Geometry: final body of the model. Coordinates: model frame, mm. Face numbers are marked on the shaded views. A direction names the side the tool comes from. Coordinates: 2 decimals unless noted, no trailing zeros. Order: outer loops, then holes, each group sorted by start corner. A loop starts at its lowest first (then second) coordinate and runs counter-clockwise, first axis right, second up. Notation, with made-up numbers: (47, -34.5) - (97, -34.5) arc R19 cw to (97, -13.5) - close; hole circle Ø1 at (62.5, -13). An arc over 180 degrees is marked (long way). Use a Markdown table: item, result. Add a question column.
```python
from build123d import *

# Parameters (mm, degrees)
F0_R     = 3.2385
F1_DEPTH = 6.35
F3_DEPTH = 4.318
F4_D     = 6.7564


with BuildPart() as f1:
    # F0 (on Top) → F1 (new body)
    with BuildSketch(Plane.XY):
        Polygon((0, -12.7), (10.9985226281, -6.35), (10.9985226281, 6.35), (0, 12.7), (-10.9985226281, 6.35), (-10.9985226281, -6.35), align=None)
        Polygon((0, 6.3204843369), (5.4737, 3.1602421685), (5.4737, -3.1602421685), (0, -6.3204843369), (-5.4737, -3.1602421685), (-5.4737, 3.1602421685), align=None, mode=Mode.SUBTRACT)
        Polygon((5.4737, -3.1602421685), (5.4737, 3.1602421685), (0, 6.3204843369), (-5.4737, 3.1602421685), (-5.4737, -3.1602421685), (0, -6.3204843369), align=None)
        Circle(F0_R, mode=Mode.SUBTRACT)
        Circle(F0_R)
    extrude(amount=F1_DEPTH)

    # F2 (on face) → F3 (cut)
    with BuildSketch(Plane.XY.offset(6.35)):
        Polygon((0, 6.3204843369), (-5.4737, 3.1602421685), (-5.4737, -3.1602421685), (0, -6.3204843369), (5.4737, -3.1602421685), (5.4737, 3.1602421685), align=None)
    extrude(amount=-F3_DEPTH, mode=Mode.SUBTRACT)

    # F4 (through all)
    with Locations(Plane(origin=(0, 0, 0), x_dir=(1, 0, 0), z_dir=(0, 0, -1))):
        with Locations((0, 0)):
            Hole(F4_D / 2)


solid = f1.part
```
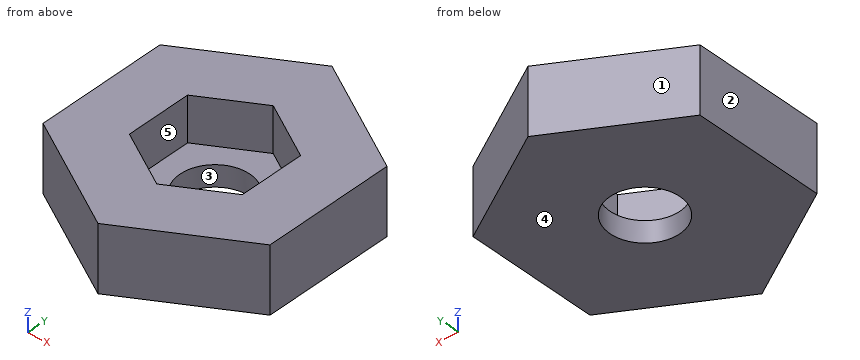
1) Set-up query: the marked faces 4 and 5. Return all of +Z, -Z, +X, -X, +Y, -Y with unobstructed straight access to the full face (end or side cutting, diameter ignored); none if empty.
2) Section C-C (x = -2). Return loops of the section in (y, z), then the cut area to 3 significant figures.
3) Section B-B (y = -2.5). Return loops of the section in (x, z).
4) Section A-A (z = 0.5). Return loops of the section in (x, y), then the cut area to 3 significant figures.
5) Pin query (flat end, axial travel): pin 1 (5.5 mm diameter, centred on x = 0, y = -0.5, fed in from +Z); pin 2 (3 mm diameter, centred on x = 4.5, y = 3, fed in from -Z); pin 3 (2 mm diameter, centred on y = -9.5, z = 3, fed in from +X). Return the tip coordinate at first contact, or that it passes through.
6) Ray query, line 1 along X through (y, z) = (4.5, 5.25); line 2 along Z through (x, y) = (1.25, -3.5); line 3 along Y through (x, z) = (-3.5, 5.5). Return the intervals inside material, ascending.
7) Draft query along Y for the marked faces 1, 2 and 3. Return one class per face: pulls with the +Y half, pulls with the -Y half, needs draft (parallel to the pull), parting line crosses it, or undercut.
8) Section D-D (z = 5). Return loops of the section in (x, y).
Values follow:
| question | item | result |
|---|---|---|
| 1 | face 4 | -Z, +X, -X, +Y, -Y |
| 1 | face 5 | +Z |
| 2 | outline | (-11.55, 0) - (-2.72, 0) - (-2.72, 2.03) - (-5.17, 2.03) - (-5.17, 6.35) - (-11.55, 6.35) - close; (2.72, 0) - (11.55, 0) - (11.55, 6.35) - (5.17, 6.35) - (5.17, 2.03) - (2.72, 2.03) - close |
| 2 | area | 90.9 mm² |
| 3 | outline | (-11, 0) - (-2.27, 0) - (-2.27, 2.03) - (-5.47, 2.03) - (-5.47, 6.35) - (-11, 6.35) - close; (2.27, 0) - (11, 0) - (11, 6.35) - (5.47, 6.35) - (5.47, 2.03) - (2.27, 2.03) - close |
| 4 | outline | (-11, -6.35) - (0, -12.7) - (11, -6.35) - (11, 6.35) - (0, 12.7) - (-11, 6.35) - close; hole circle Ø6.76 at (0, 0) |
| 4 | area | 383 mm² |
| 5 | pin 1 | passes through |
| 5 | pin 2 | stops at z = 0 |
| 5 | pin 3 | stops at x = 7.27 |
| 6 | line 1 | x = -11 to -3.15, 3.15 to 11 |
| 6 | line 2 | z = 0 to 2.03 |
| 6 | line 3 | y = -10.68 to -4.3, 4.3 to 10.68 |
| 7 | face 1 | pulls with the +Y half |
| 7 | face 2 | needs draft |
| 7 | face 3 | undercut |
| 8 | outline | (-11, -6.35) - (0, -12.7) - (11, -6.35) - (11, 6.35) - (0, 12.7) - (-11, 6.35) - close; hole (-5.47, -3.16) - (0, -6.32) - (5.47, -3.16) - (5.47, 3.16) - (0, 6.32) - (-5.47, 3.16) - close |
